Autodesk Inventor part; units mm, degrees
ref_plane "YZ Plane" through (0, 0, 0) normal (1, 0, 0) x (0, 1, 0)
ref_plane "XZ Plane" through (0, 0, 0) normal (0, 1, 0) x (-1, 0, 0)
ref_plane "XY Plane" through (0, 0, 0) normal (0, 0, 1) x (1, 0, 0)
sketch "Náčrt1" plane through (0, 0, 0) normal (0, 0, 1) x (1, 0, 0)
  line L0 (0, -50) -> (50, -50)
  line L1 (50, -50) -> (50, 50)
  line L2 (50, 50) -> (0, 50)
  line L3 (0, 50) -> (0, -50)
  point P0 (0, 0)
  point P1 (50, 0)
  point P2 (0, 0)
  dimension "d0" = 50
  dimension "d1" = 100
extrude "Vysunutí1" add sketch "Náčrt1" along normal blind 3
sketch "Náčrt2" plane through (50, -50, 0) normal (1, 0, 0) x (0, 0, -1)
  line L0 (0, 0) -> (0, 100)
  line L1 (0, 100) -> (-30, 86.0108)
  line L2 (-30, 86.0108) -> (-30, 83.804)
  line L3 (-30, 83.804) -> (0, 97.7932)
  line L4 (-3, 0) -> (-3, 100)
  line L5 (0, 100) -> (-3, 100)
  point P0 (0, 50)
  point P1 (-3, 98.6011)
  dimension "d4" = 65
  dimension "d6" = 2
  dimension "d7" = 30
extrude "Vysunutí2" add sketch "Náčrt2" against normal up to surface (50 mm away) contours L3 L4 L1 L0 | L3 L2 L1 L4
extrude "Vysunutí3" cut sketch "Náčrt2" against normal through all contours L1 L4 L5
ref_plane "Pracovní rovina1" through (50, 50, 0) normal (0, -1, 0) x (1, 0, 0)
mirror "Zrcadlit1" about plane through (0, 0, 0) normal (1, 0, 0)
sketch "Náčrt3" plane through (50, 50, 0) normal (0, -1, 0) x (1, 0, 0)
  line L0 (-12.748, 22.13) -> (-21.41, 22.13)
  line L1 (-21.41, 22.13) -> (-21.41, 8.58)
  line L2 (-21.41, 8.58) -> (-12.748, 8.58)
  line L3 (-12.748, 8.58) -> (-12.748, 22.13)
  line L4 (-54.03, 8.58) -> (-43.38, 8.58)
  line L5 (-43.38, 8.58) -> (-43.38, 22.13)
  line L6 (-43.38, 22.13) -> (-54.03, 22.13)
  line L7 (-54.03, 22.13) -> (-54.03, 8.58)
  line L8 (0, 0) -> (0, 30)
  line L9 (0, 0) -> (-50, 0)
  line L10 (-79.1, 22.13) -> (-87.762, 22.13)
  line L11 (-87.762, 22.13) -> (-87.762, 8.58)
  line L12 (-87.762, 8.58) -> (-79.1, 8.58)
  line L13 (-79.1, 8.58) -> (-79.1, 22.13)
  line L14 (-100, 0) -> (-100, 30)
  line L15 (-87.762, 22.13) -> (-100, 22.13)
  line L16 (-87.762, 8.58) -> (-100, 8.58)
  line L17 (-12.748, 22.13) -> (0, 22.13)
  line L18 (-12.748, 8.58) -> (0, 8.58)
  dimension "d13" = 22.13
  dimension "d14" = 21.97
  dimension "d15" = 8.662
  dimension "d18" = 25.07
  dimension "d19" = 12.238
  dimension "d20" = 10.65
  dimension "d21" = 8.662
  dimension "d22" = 8.58
extrude "Vysunutí4" cut sketch "Náčrt3" along normal through all
properties part number "Test rampy"
Input: part model. Units: mm. Frame: model coordinates. A direction names the side the tool comes from. Round coordinates to 2 decimals unless told otherwise and drop trailing zeros. Loops run counter-clockwise (first coordinate to the right, second up) from the corner with the lowest first, then second, coordinate; pieces in that order, holes last. Notation, with made-up numbers: (70.5, -33) -> (111.5, -33) arc R18 ccw to (111.5, -21) -> close; hole circle Ø7 at (-24.75, 35). An arc over 180 degrees is marked (long way). One line per item, written item: value.
(1) Pin query (flat end, axial travel): pin 1 (4.5 mm diameter, centred on y = 43, z = 12, fed in from -X); pin 2 (2.5 mm diameter, centred on y = 42, z = 15.5, fed in from +X); pin 3 (1.8 mm diameter, centred on x = -37, y = 44.5, fed in from +Z); pin 4 (1.1 mm diameter, centred on x = -36.5, y = 38, fed in from -Z). Return the tip coordinate at first contact, or that it passes through.
Geometry check:
pin 1: x = -29.1
pin 2: x = 28.59
pin 3: z = 8.58
pin 4: z = 0
(2) Mould query, pull axis Z, two halves, no side actions, for faces 5 (the face through (-1, -50, 1)), 6 (the face through (0.7, 46.212, 8.123)), 7 (the face through (1, 39, 22.13)). Classes: pulls with the +Z half, pulls with the -Z half, needs draft (parallel to the pull), parting line crosses it, or undercut.
Geometry check:
face 5: needs draft
face 6: pulls with the +Z half
face 7: undercut
(3) Section B-B (z = 18.25). Return the cut outline in (x, y), plus the area to 3 significant figures.
Geometry check:
outline: (-29.1, 39.28) -> (-4.03, 39.28) -> (-4.03, 41.49) -> (-29.1, 41.49) -> close; (6.62, 39.28) -> (28.59, 39.28) -> (28.59, 41.49) -> (6.62, 41.49) -> close
area: 104 mm2
(4) Section D-D (y = -4.5). Return the cut outline in (x, z), plus the area to 3 significant figures.
Geometry check:
outline: (-50, 0) -> (50, 0) -> (50, 3) -> (-50, 3) -> close
area: 300 mm2
(5) Section C-C (x = 26). Return the cut outline in (y, z).
Geometry check:
outline: (-50, 0) -> (50, 0) -> (36.01, 30) -> (33.8, 30) -> (46.39, 3) -> (-50, 3) -> close
(6) Section A-A (x = 1.5). Return the cut outline in (y, z).
Geometry check:
outline: (-50, 0) -> (50, 0) -> (46, 8.58) -> (43.79, 8.58) -> (46.39, 3) -> (-50, 3) -> close; (33.8, 30) -> (37.47, 22.13) -> (39.68, 22.13) -> (36.01, 30) -> close
(7) Material intervals for line 1 (Z direction, x = -43, y = 6); line 2 (Z direction, x = 9, y = 43); line 3 (Z direction, x = -38.5, y = 39.5), sorted ascending. Write a range as [from, to].
Geometry check:
line 1: [0, 3]
line 2: [0, 3], [10.28, 15.01]
line 3: [0, 3], [22.13, 22.52]
(8) Set-up query: faces 1 (the face through (-4.03, 42, 15)), 2 (the face through (39, 39, 22.13)), 3 (the face through (1, 45, 8.58)), 4 (the face through (-39, 39, 22.13)). Return all of +Z, -Z, +X, -X, +Y, -Y with unobstructed straight access to the full face (end or side cutting, diameter ignored); none if empty.
Geometry check:
face 1: +Y, -Y
face 2: +X, +Y, -Y
face 3: +Z, +Y, -Y
face 4: -X, +Y, -Y
